from build123d import *

# Parameters (mm, degrees)
DI_METRO_DE_TALADRO_1_4_0_25_1_D = 6.35


with BuildPart() as part:
    # Croquis1 → Revolución1 (revolve)
    with BuildSketch(Plane.XY, mode=Mode.PRIVATE) as revoluci_n1_sk:
        Polygon((-9.525, 0), (0, 0), (0, 50.038), (-9.525, 50.038), (-9.525, 44.86275), (-4.525, 44.86275), (-2.73, 43.06775), (-2.73, 38.71775), (-4.525, 36.92275), (-9.525, 36.92275), (-9.525, 22.63475), (-9.525, 2), align=None)
    revolve(revoluci_n1_sk.sketch.rotate(Axis((0, 0, 0), (0, 1, 0)), 270), axis=Axis((0, 0, 0), (0, 1, 0)))

    # Diámetro de taladro 1/4 (0.25)1 (through all)
    with Locations(Plane(origin=(0, 17.875, 9.525), x_dir=(1, 0, 0), z_dir=(0, 0, 1))):
        with Locations((0, 0)):
            Hole(DI_METRO_DE_TALADRO_1_4_0_25_1_D / 2)


solid = part.part
Check sheet for the modelled part. Datum: model origin and axes. Units: mm. A direction names the side the tool comes from. Round coordinates to 2 decimals unless told otherwise and drop trailing zeros. Loops run counter-clockwise (first coordinate to the right, second up) from the corner with the lowest first, then second, coordinate; pieces in that order, holes last. Notation, with made-up numbers: (26.25, 80) -> (62.25, 80) arc R28 cw to (62.25, 98) -> close; hole circle Ø1 at (24, -4). An arc over 180 degrees is marked (long way). Put each result on its own line as item: value. Start each with the question number.
1. Section check B-B (z = 7.75). Enter the section's corners in (x, y) (3 decimals), plus the area to 3 significant figures.
2. Section check C-C (z = 0). Enter the section's corners in (x, y) (3 decimals), plus the area to 3 significant figures.
3. Access from +Z, -Z, +X, -X, +Y, -Y to the whole of each face (thin tool, end or side, straight path). Record for faces 1 (the face through (-2.3, 36.923, 4.1)), 2 (the face through (0.413, 21.023, -0.13)).
4. Gauge pin test, flat ends, axial feed: pin 1 (5.5 mm diameter, centred on x = 0, y = 17.875, fed in from +Z); pin 2 (1.5 mm diameter, centred on x = -3, y = 38, fed in from -Z). Record the tip position at first contact, or that the pin passes through.
5. Scan lines: probe 1 along Y at (x, z) = (0, 5); probe 2 along Y at (x, z) = (0, -0.25); probe 3 along Y at (x, z) = (7.25, 2). Record each from-to range of solid material in increasing order.
6. Section check D-D (y = 28). Enter the section's corners in (x, z) (3 decimals).
7. Section check A-A (x = 0). Enter the section's corners in (y, z) (3 decimals).
8. Draft check along Y on faces 3 (the face through (2.77, 38.61, 0.62)), 4 (the face through (0, 50.038, 0)), 5 (the face through (5.796, 47.414, 7.559)). Enter one of: +Y half, -Y half, draft (parallel to the pull), parting line (faces both ways), or undercut.
Findings:
1. outline: (-5.537, 0) -> (5.537, 0) -> (5.537, 36.923) -> (-5.537, 36.923) -> close; (-5.537, 44.863) -> (5.537, 44.863) -> (5.537, 50.038) -> (-5.537, 50.038) -> close; hole circle Ø6.35 at (0, 17.875)
1. area: 435 mm^2
2. outline: (-9.525, 0) -> (9.525, 0) -> (9.525, 36.923) -> (4.525, 36.923) -> (2.73, 38.718) -> (2.73, 43.068) -> (4.525, 44.863) -> (9.525, 44.863) -> (9.525, 50.038) -> (-9.525, 50.038) -> (-9.525, 44.863) -> (-4.525, 44.863) -> (-2.73, 43.068) -> (-2.73, 38.718) -> (-4.525, 36.923) -> (-9.525, 36.923) -> close; hole circle Ø6.35 at (0, 17.875)
2. area: 820 mm^2
3. face 1: none
3. face 2: +Z, -Z
4. pin 1: passes through
4. pin 2: stops at z = -3.15
5. probe 1: y = 0 to 14.7, 21.05 to 36.92, 44.86 to 50.04
5. probe 2: y = 0 to 14.7, 21.05 to 50.04
5. probe 3: y = 0 to 36.92, 44.86 to 50.04
6. outline: circle Ø19.05 at (0, 0)
7. outline: (0, -9.525) -> (14.7, -9.525) -> (14.7, 9.525) -> (0, 9.525) -> close; (21.05, -9.525) -> (36.923, -9.525) -> (36.923, -4.525) -> (38.718, -2.73) -> (43.068, -2.73) -> (44.863, -4.525) -> (44.863, -9.525) -> (50.038, -9.525) -> (50.038, 9.525) -> (44.863, 9.525) -> (44.863, 4.525) -> (43.068, 2.73) -> (38.718, 2.73) -> (36.923, 4.525) -> (36.923, 9.525) -> (21.05, 9.525) -> close
8. face 3: undercut
8. face 4: +Y half
8. face 5: draft
